from build123d import *

# Parameters (mm, degrees)
F0_R     = 1.75
F0_R_2   = 2
F1_DEPTH = 5
F2_DEPTH = 7.5
F3_DEPTH = 2.5
F4_R     = 1.65
F5_DEPTH = 29.75
F6_R     = 4.99999


# Not quite as in the source:
# - a fillet or chamfer is up to 0.001 mm smaller than in the source, because OpenCascade refuses the exact size


with BuildPart() as f1:
    # F0 (on Top) → F1 (new body)
    with BuildSketch(Plane.XY):
        with BuildLine():
            Line((-5, 10), (-8, 10))
            Line((-8, 10), (-8, -15))
            Line((-8, -15), (0, -15))
            ThreePointArc((0, -15), (3.5355339059, -13.5355339059), (5, -10))
            Line((5, -10), (5, 10))
            ThreePointArc((5, 10), (0, 15), (-5, 10))
        make_face()
        with Locations((0, -10)):
            Circle(F0_R, mode=Mode.SUBTRACT)
        with Locations((0, 10)):
            Circle(F0_R_2, mode=Mode.SUBTRACT)
    extrude(amount=F1_DEPTH)

    # F0 (on Top) → F2 (join)
    with BuildSketch(Plane.XY):
        Polygon((-8, 10), (-18, 10), (-18, -19.75), (-8, -19.75), (-8, -15), align=None)
    extrude(amount=F2_DEPTH)

    # F0 (on Top) → F3 (join)
    with BuildSketch(Plane.XY):
        Polygon((-8, 10), (-18, 10), (-18, -19.75), (-8, -19.75), (-8, -15), align=None)
    extrude(amount=-F3_DEPTH)

    # F4 (on face) → F5 (cut, through all)
    with BuildSketch(Plane.XZ.offset(19.75)):
        with Locations((-13, 2.5)):
            Circle(F4_R)
    extrude(amount=-F5_DEPTH, mode=Mode.SUBTRACT)

    # F6 (radius 5 in the source; OpenCascade refuses exactly that, so slightly less here)
    f6_edges = [f1.edges().sort_by_distance(p)[0] for p in [
        (-18, -4.875, 7.5),
        (-18, -4.875, -2.5),
        (-8, -4.875, 7.5),
        (-8, -4.875, -2.5),
    ]]
    fillet(f6_edges, radius=F6_R)


solid = f1.part
Geometry check sheet. Reference: the model listing, model coordinates, mm. A direction names the side the tool comes from. Round coordinates to 2 decimals unless told otherwise and drop trailing zeros. Write each loop counter-clockwise with the first axis right and the second up, starting at its lowest first coordinate (ties: lowest second). Pieces come first, ordered by that corner, then holes.
Item 1: Mould release check, pull along Y, two halves, no side actions. Record for faces 6 (the face through (-11.426, -5.083, 2.996)), 7 (the face through (3, -14, 2)), 8 (the face through (0, 12, 2)), 9 (the face through (0, 15, 2)): +Y half, -Y half, draft (parallel to the pull), parting line (faces both ways), or undercut.
Determined:
face 6: draft
face 7: -Y half
face 8: undercut
face 9: +Y half
Item 2: Go/stop test with flat-tipped pins: pin 1 Ø4.5 at (x, y) = (0, 10) entering from +Z; pin 2 Ø5 at (x, y) = (2, -13) entering from -Z; pin 3 Ø2 at (x, y) = (-11.5, -0.5) entering from -Z. Record where each tip stops, or that it passes through.
Determined:
pin 1: stops at z = 5
pin 2: stops at z = 0
pin 3: stops at z = -2.47
Item 3: Access from +Z, -Z, +X, -X, +Y, -Y to the whole of each face (thin tool, end or side, straight path). Record for faces 1 (the face through (-2, 0, 0)), 2 (the face through (-2, 0, 5)), 3 (the face through (-16.5, -5.08, -1.07)), 4 (the face through (-11, 10, 1)), 5 (the face through (-16.57, -5.08, 6)).
Determined:
face 1: -Z, +X, +Y, -Y
face 2: +Z, +X, +Y, -Y
face 3: -Z, -X, +Y, -Y
face 4: +Z, -Z, -X, +Y
face 5: +Z, -X, +Y, -Y
Item 4: Section check C-C (x = -0.75). Record the boundary of the cut face in (y, z), plus the area to 3 significant figures.
Determined:
outline: (-15, 0) - (-11.58, 0) - (-11.58, 5) - (-15, 5) - close; (-8.42, 0) - (8.15, 0) - (8.15, 5) - (-8.42, 5) - close; (11.85, 0) - (14.94, 0) - (14.94, 5) - (11.85, 5) - close
area: 115 mm2
Item 5: Material ranges on line 1 along Z through (x, y) = (-13, -9.5); line 2 along Z through (x, y) = (-5.75, 9); line 3 along Y through (x, z) = (-9.75, 6.25), recorded low to high.
Determined:
line 1: z = -2.5 to 0.85, 4.15 to 7.5
line 2: z = 0 to 5
line 3: y = -19.75 to 10
Item 6: Section check A-A (y = 9.5). Give the number of separate pieces and of enclosed holes in the cut face, plus the area to 3 significant figures.
Determined:
separate pieces: 2
enclosed holes: 1
area: 117 mm2
